Part print with two shaded views. Sizes in mm from the minimum x, y, z corner. A direction names the side the tool comes from. Coordinates: 2 decimals unless noted, no trailing zeros. Loops run counter-clockwise (first coordinate to the right, second up) from the corner with the lowest first, then second, coordinate; pieces in that order, holes last. Notation, with made-up numbers: (46.25, 63) -> (56.25, 63) arc R31 ccw to (56.25, 93) -> close; hole circle Ø3 at (-7, 7). An arc over 180 degrees is marked (long way). Return JSON: item names as keys, results as strings. Group by question number.
(1) Mould opens along X. For the marked faces 4, 5 and 6 say: pulls with the +X half, pulls with the -X half, needs draft (parallel to the pull), parting line crosses it, or undercut.
(2) Tool access for the marked faces 1, 2 and 3: list every direction of +Z, -Z, +X, -X, +Y, -Y with a clear straight run to the whole face (end or side of a thin tool).
(3) Probe L1, parallel to X at y = 38.5, z = 6; L2, parallel to X at y = 30, z = 42; L3, parallel to Z at x = 34, y = 11. List the from-to ranges inside material, lowest first.
(4) Saw through at C-C on x = 8. Write the cut outline in (y, z), then the cut area to 3 significant figures.
(5) Flat gauge pins, fed straight in: pin 1 Ø8 at (x, y) = (50, 13) entering from -Z; pin 2 Ø2.5 at (x, y) = (2, 11) entering from +Z; pin 3 Ø11 at (x, y) = (17, 15) entering from +Z. Where does each tip first touch, or does it go through?
(6) Saw through at D-D on z = 21. Write the cut outline in (x, y).
(7) Saw through at B-B on y = 33. Write the cut outline in (x, z), then the cut area to 3 significant figures.
(8) Saw through at A-A on z = 34.5. Write the cut outline in (x, y), then the cut area to 3 significant figures.
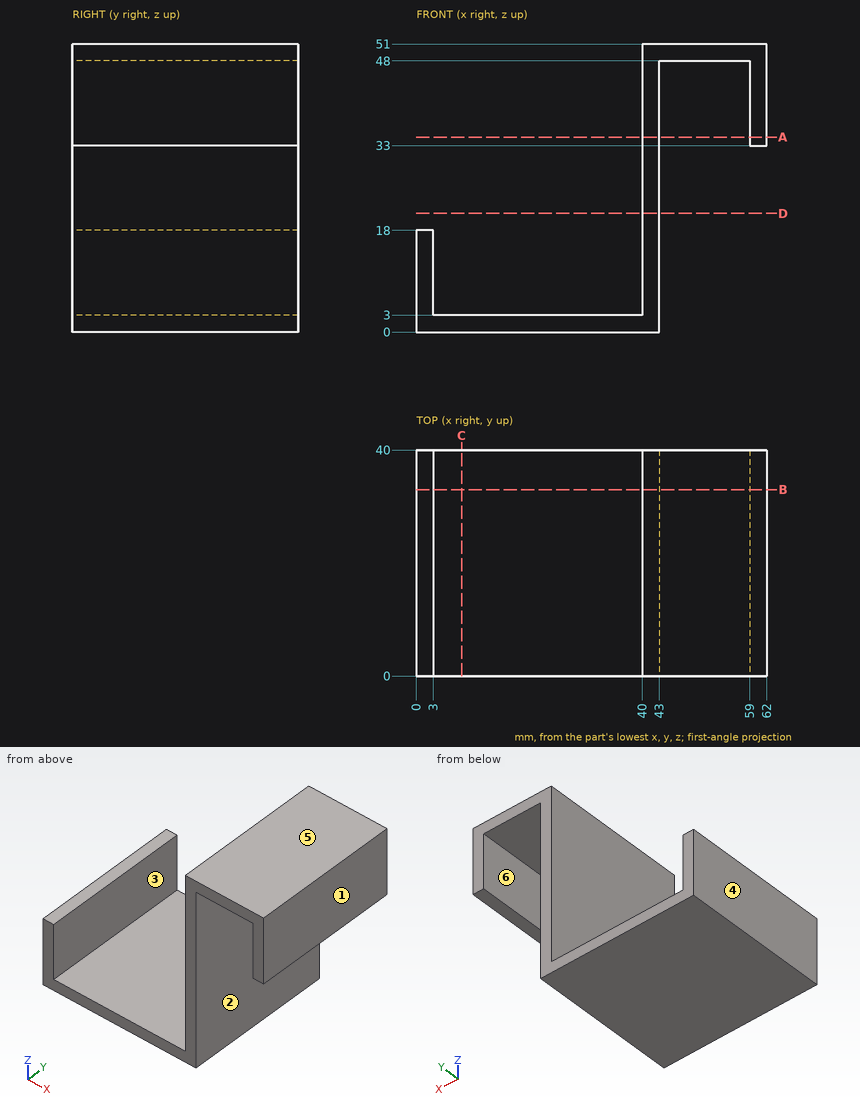
Geometry results:
{
 "1": {"face 4": "pulls with the -X half", "face 5": "needs draft", "face 6": "undercut"},
 "2": {"face 1": "+Z, -Z, +X, +Y, -Y", "face 2": "-Z, +Y, -Y", "face 3": "+Z, +Y, -Y"},
 "3": {"L1": "0 to 3, 40 to 43", "L2": "40 to 43, 59 to 62", "L3": "0 to 3"},
 "4": {"outline": "(0, 0) -> (40, 0) -> (40, 3) -> (0, 3) -> close", "area": "120 mm²"},
 "5": {"pin 1": "z = 48", "pin 2": "z = 18", "pin 3": "z = 3"},
 "6": {"outline": "(40, 0) -> (43, 0) -> (43, 40) -> (40, 40) -> close"},
 "7": {"outline": "(0, 0) -> (43, 0) -> (43, 48) -> (59, 48) -> (59, 33) -> (62, 33) -> (62, 51) -> (40, 51) -> (40, 3) -> (3, 3) -> (3, 18) -> (0, 18) -> close", "area": "420 mm²"},
 "8": {"outline": "(40, 0) -> (43, 0) -> (43, 40) -> (40, 40) -> close; (59, 0) -> (62, 0) -> (62, 40) -> (59, 40) -> close", "area": "240 mm²"}
}
